The listing builds one solid part. Answer for the finished solid, in the listing's coordinates (mm). A direction names the side the tool comes from. Coordinates: 2 decimals unless noted, no trailing zeros. Order: outer loops, then holes, each group sorted by start corner. A loop starts at its lowest first (then second) coordinate and runs counter-clockwise, first axis right, second up. Notation, with made-up numbers: M 34.5,52 L 80.5,52 A25 cw 80.5,71 Z; hole C 83.5,76 d3. An arc over 180 degrees is marked long. One line per item, written item: value. Start each with the question number.
Q1. For faces 1 (the flat face through (17, 23, 12.7)), 2 (the flat face through (-1, 1, 0)), determine the directions among +Z, -Z, +X, -X, +Y, -Y from which every point of the face is accessible in a straight line to the end or side of a thin tool.
Q2. The part is cut by section D-D on x = -28. Give the vertices of the cut face in (y, z), then the cut area to 3 significant figures.
Q3. Straight lines are drawn through the part: line 1 along X through (y, z) = (-7, 22); line 2 along Y through (x, z) = (0, 18.75) (3 decimals); line 3 along X through (y, z) = (-28.5, 12.75). For each, find the intervals that lie inside material, in ascending order. Write a range as [from, to].
Q4. Determine the mould class of faces 3 (the flat face through (-1, -38.1, 13)), 4 (the flat face through (38.1, -1, 13)), 5 (the cylindrical face through (29.29, -14.82, 19.14)) for opening direction X: pulls with the +X half, pulls with the -X half, needs draft (parallel to the pull), parting line crosses it, or undercut.
Q5. The part is cut by section C-C on z = 18.5. Give the vertices of the cut face in (x, y) (3 decimals), then the cut area to 3 significant figures.
Q6. This flat-tipped pin is pushed along its axis until it touches: pin 1 Ø6.5 at (x, y) = (28, -8) entering from +Z. Where does it stop, or does it pass through?
Q7. The part is cut by section A-A on x = 0. Give the vertices of the cut face in (y, z) (3 decimals).
Q8. The part is cut by section B-B on y = -5. Give the vertices of the cut face in (x, z), then the cut area to 3 significant figures.
```python
from build123d import *

# Parameters (mm, degrees)
F0_W            = 76.2
F0_H            = 76.2
F1_DEPTH        = 25.4
F2_R            = 6.35
F3_DEPTH        = 12.7
F3_COPIES_COUNT = 5


# Not quite as in the source:
# - a pattern or mirror of a feature is missing from the dataset's text; its kind, count and spacing are read off the source's solid


with BuildPart() as f1:
    # F0 (on Top) → F1 (new body)
    with BuildSketch(Plane.XY):
        Rectangle(F0_W, F0_H)
    extrude(amount=F1_DEPTH)

    # F2 (on face) → F3 (cut)
    with BuildSketch(Plane.XY.offset(25.4)):
        with Locations((0, -28.575)):
            Circle(F2_R)
    f3 = extrude(amount=-F3_DEPTH, mode=Mode.SUBTRACT)

    # F3_copies: F3 ×5 about axis
    f3_copies_axis = Axis((0, 0, 0), (0, 0, 1))
    for i in range(1, F3_COPIES_COUNT):
        add(f3.rotate(f3_copies_axis, i * 360 / F3_COPIES_COUNT), mode=Mode.SUBTRACT)


solid = f1.part
```
Output:
1. face 1: +Z
1. face 2: -Z, +X, -X, +Y, -Y
2. outline: M -38.1,0 L 38.1,0 L 38.1,25.4 L -2.53,25.4 L -2.53,12.7 L -15.13,12.7 L -15.13,25.4 L -38.1,25.4 Z
2. area: 1,780 mm^2
3. line 1: x = [-38.1, -33.26], [-21.1, 21.1], [33.26, 38.1]
3. line 2: y = [-38.1, -34.925], [-22.225, 38.1]
3. line 3: x = [-38.1, -6.35], [6.35, 38.1]
4. face 3: needs draft
4. face 4: pulls with the +X half
4. face 5: undercut
5. outline: M -38.1,-38.1 L 38.1,-38.1 L 38.1,38.1 L -38.1,38.1 Z; hole C -27.176,-8.83 d12.7; hole C -16.796,23.118 d12.7; hole C 0,-28.575 d12.7; hole C 16.796,23.118 d12.7; hole C 27.176,-8.83 d12.7
5. area: 5,170 mm^2
6. pin 1: stops at z = 12.7
7. outline: M -38.1,0 L 38.1,0 L 38.1,25.4 L -22.225,25.4 L -22.225,12.7 L -34.925,12.7 L -34.925,25.4 L -38.1,25.4 Z
8. outline: M -38.1,0 L 38.1,0 L 38.1,25.4 L 32.24,25.4 L 32.24,12.7 L 22.11,12.7 L 22.11,25.4 L -22.11,25.4 L -22.11,12.7 L -32.24,12.7 L -32.24,25.4 L -38.1,25.4 Z
8. area: 1,680 mm^2
